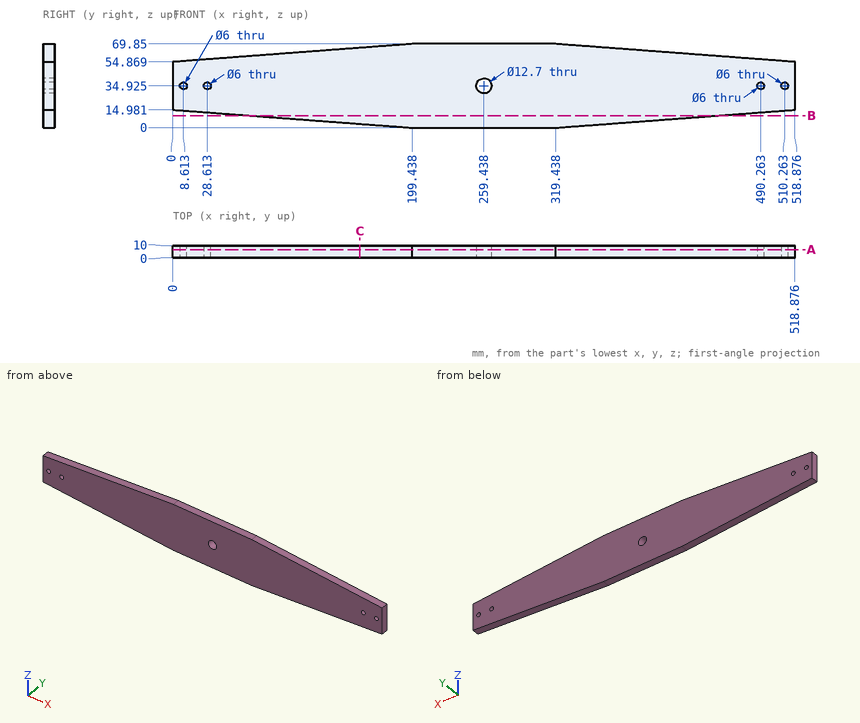
Job drawing, mm, ordinate dimensions from the low corner. One solid piece. Round coordinates to 2 decimals unless told otherwise and drop trailing zeros. Write each loop counter-clockwise with the first axis right and the second up, starting at its lowest first coordinate (ties: lowest second). Pieces come first, ordered by that corner, then holes. Notation, with made-up numbers: M 40,24.5 L 64,24.5 A11 cw 64,45.5 Z; hole C 49.25,73.5 d6. An arc over 180 degrees is marked long. Return JSON: item names as keys, results as strings. Group by question number.
(1) Saw through at A-A on y = 6.75. Count the separate pieces of the cut face and the enclosed holes in it, then the cut area to 3 significant figures.
(2) Pin check, flat tips, straight feed: pin 1 Ø5 at (y, z) = (2.5, 49.5) entering from -X; pin 2 Ø1 at (x, y) = (400.5, 1.5) entering from -Z; pin 3 Ø1.5 at (x, y) = (425.5, 5.5) entering from +Z. Stop position of each tip, or through.
(3) Drill centre lines: probe 1 along X at (y, z) = (8, 30.5) (1 decimal); probe 2 along Z at (x, y) = (409.5, 8.5) (1 decimal); probe 3 along Z at (x, y) = (442.5, 7.5). Where is each one in solid material? Low to high.
(4) Saw through at B-B on z = 10. Write the cut outline in (x, y).
(5) Saw through at C-C on x = 156. Write the cut outline in (y, z), then the cut area to 3 significant figures.
Returned:
{
 "1": {"separate pieces": "1", "enclosed holes": "5", "area": "30,000 mm²"},
 "2": {"pin 1": "x = 0", "pin 2": "z = 6.05", "pin 3": "z = 61.94"},
 "3": {"probe 1": "0 to 254.9, 264 to 518.9", "probe 2": "6.8 to 63.1", "probe 3": "9.24 to 60.61"},
 "4": {"outline": "M 66.31,0 L 452.56,0 L 452.56,10 L 66.31,10 Z"},
 "5": {"outline": "M 0,3.26 L 10,3.26 L 10,66.59 L 0,66.59 Z", "area": "633 mm²"}
}
